Geometry check sheet. Reference: drawing and pictorial views, mm from the part's lowest x, y, z. A direction names the side the tool comes from. Round coordinates to 2 decimals unless told otherwise and drop trailing zeros. Order: outer loops, then holes, each group sorted by start corner. A loop starts at its lowest first (then second) coordinate and runs counter-clockwise, first axis right, second up.
Q1. Cross-section at A-A on z = 12. Record the cut outline in (x, y).
Q2. Cross-section at C-C on x = 25. Record the cut outline in (y, z).
Q3. Set-up check for the marked faces 1, 2, 3 and 4: record each of +Z, -Z, +X, -X, +Y, -Y from which the full face is reachable in a straight line by a thin tool's end or side.
Q4. Depth check by flat-ended pin: P1, Ø5, axis at x = 7.5, y = 59, coming from the +Z side; P2, Ø6, axis at y = 10, z = 12, coming from the -X side; P3, Ø8.5, axis at x = 24.5, y = 21, coming from the -Z side. Enter the tip coordinate at first touch or a pass-through.
Q5. Cross-section at B-B on y = 61. Record the cut outline in (x, z), then the cut area to 3 significant figures.
Q6. Scan lines: probe 1 along Y at (x, z) = (10.5, 4); probe 2 along Y at (x, z) = (25, 21); probe 3 along Y at (x, z) = (7, 9). Record each from-to range of solid material in increasing order.
Q7. Cross-section at D-D on y = 10. Record the cut outline in (x, z).
Q8. Mould release check, pull along X, two halves, no side actions. Record for the marked faces 5, 6 and 7: +X half, -X half, draft (parallel to the pull), parting line (faces both ways), or undercut.
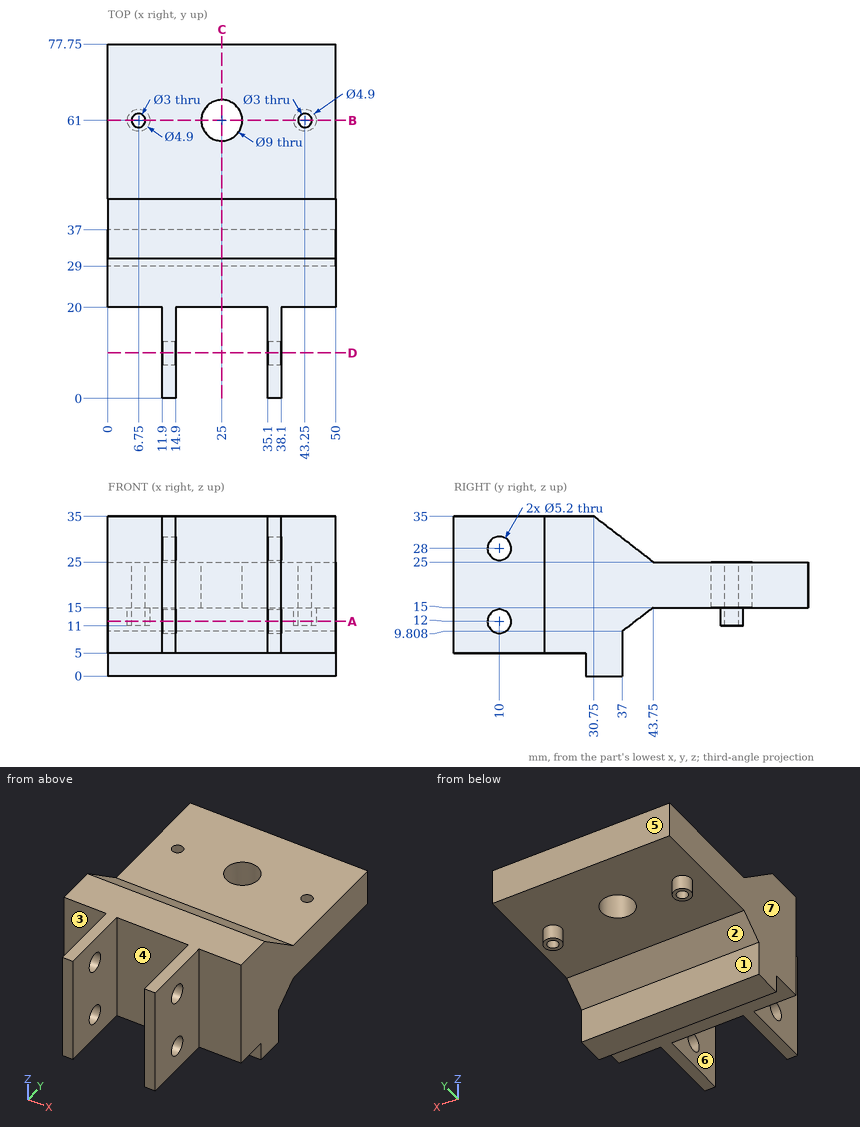
Results found:
1. outline: (0, 20) - (11.9, 20) - (11.9, 12.6) - (14.9, 12.6) - (14.9, 20) - (35.1, 20) - (35.1, 12.6) - (38.1, 12.6) - (38.1, 20) - (50, 20) - (50, 39.85) - (0, 39.85) - close; circle Ø4.9 at (6.75, 61); (11.9, 0) - (14.9, 0) - (14.9, 7.4) - (11.9, 7.4) - close; (35.1, 0) - (38.1, 0) - (38.1, 7.4) - (35.1, 7.4) - close; circle Ø4.9 at (43.25, 61); hole circle Ø3 at (6.75, 61); hole circle Ø3 at (43.25, 61)
2. outline: (20, 5) - (29, 5) - (29, 0) - (37, 0) - (37, 9.81) - (43.75, 15) - (56.5, 15) - (56.5, 25) - (43.75, 25) - (30.75, 35) - (20, 35) - close; (65.5, 15) - (77.75, 15) - (77.75, 25) - (65.5, 25) - close
3. face 1: -Z, +X, -X, +Y
3. face 2: -Z, +X, -X
3. face 3: +Z, -Z, -X, -Y
3. face 4: +Z, -Z, -Y
4. P1: stops at z = 25
4. P2: stops at x = 11.9
4. P3: stops at z = 5
5. outline: (0, 15) - (4.3, 15) - (4.3, 11) - (5.25, 11) - (5.25, 25) - (0, 25) - close; (8.25, 11) - (9.2, 11) - (9.2, 15) - (20.5, 15) - (20.5, 25) - (8.25, 25) - close; (29.5, 15) - (40.8, 15) - (40.8, 11) - (41.75, 11) - (41.75, 25) - (29.5, 25) - close; (44.75, 11) - (45.7, 11) - (45.7, 15) - (50, 15) - (50, 25) - (44.75, 25) - close
5. area: 365 mm2
6. probe 1: y = 29 to 37
6. probe 2: y = 20 to 56.5, 65.5 to 77.75
6. probe 3: y = 20 to 37
7. outline: (11.9, 5) - (14.9, 5) - (14.9, 9.4) - (11.9, 9.4) - close; (11.9, 14.6) - (14.9, 14.6) - (14.9, 25.4) - (11.9, 25.4) - close; (11.9, 30.6) - (14.9, 30.6) - (14.9, 35) - (11.9, 35) - close; (35.1, 5) - (38.1, 5) - (38.1, 9.4) - (35.1, 9.4) - close; (35.1, 14.6) - (38.1, 14.6) - (38.1, 25.4) - (35.1, 25.4) - close; (35.1, 30.6) - (38.1, 30.6) - (38.1, 35) - (35.1, 35) - close
8. face 5: draft
8. face 6: undercut
8. face 7: -X half
